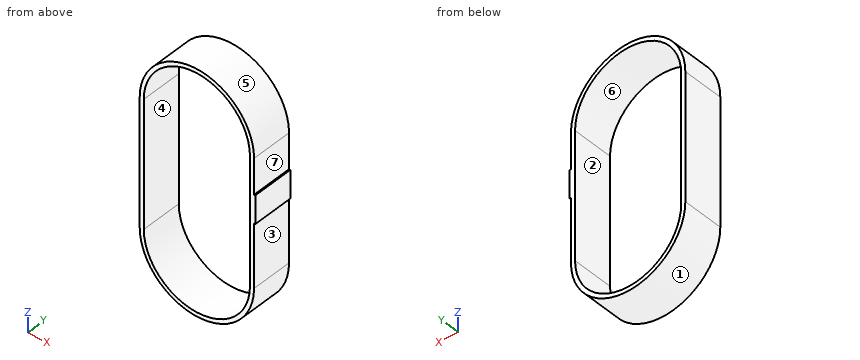
```python
from build123d import *

# Parameters (mm, degrees)
F1_DEPTH = 25.4
F2_T     = -2.54
F3_W     = 25.4
F3_H     = 17.367277
F4_DEPTH = 0.7874


with BuildPart() as f1:
    # F0 (on Front) → F1 (new body)
    with BuildSketch(Plane.XZ):
        with BuildLine():
            ThreePointArc((17.045487, 22.002723), (-18.514513, 57.562723), (-54.074513, 22.002723))
            Line((-54.074513, 22.002723), (-54.074513, -56.737277))
            ThreePointArc((-54.074513, -56.737277), (-18.514513, -92.297277), (17.045487, -56.737277))
            Line((17.045487, -56.737277), (17.045487, 22.002723))
        make_face()
    extrude(amount=F1_DEPTH)

    # F2
    f2_openings = [f1.faces().sort_by_distance(p)[0] for p in [
        (-18.514513, -25.4, -17.367277),
        (-18.514513, 0, -17.367277),
    ]]
    offset(amount=F2_T, openings=f2_openings)

    # F3 (on face) → F4 (join)
    with BuildSketch(Plane.YZ.offset(17.045487)):
        with Locations((-12.7, -8.683638)):
            Rectangle(F3_W, F3_H)
    extrude(amount=F4_DEPTH)


solid = f1.part
```
Here's how the part is built. I have some questions about the finished solid (model axes, mm). Face numbers are marked on the shaded views. A direction names the side the tool comes from. Coordinates: 2 decimals unless noted, no trailing zeros. Loops run counter-clockwise (first coordinate to the right, second up) from the corner with the lowest first, then second, coordinate; pieces in that order, holes last. Notation, with made-up numbers: (35, -25) -> (52, -25) arc R15 cw to (52, -4) -> close; hole circle Ø9 at (82.25, 28). An arc over 180 degrees is marked (long way). Return JSON: item names as keys, results as strings.
1) Will these pins go through, and if not, where does the flat tip stop? pin 1 (4 mm diameter, centred on x = -13.5, y = -23, fed in from +Z); pin 2 (12 mm diameter, centred on y = -21.5, z = -27.5, fed in from +X); pin 3 (3 mm diameter, centred on x = -33, y = -12, fed in from +Z).
Results below:
{"pin 1": "z = 57.43", "pin 2": "x = 17.05", "pin 3": "z = 55.11"}
2) If we section it at C-C, the plane x = -18.5: Write out the boundary of the cut face in (y, z), then the cut area to 3 significant figures.
Results below:
{"outline": "(-25.4, -92.3) -> (0, -92.3) -> (0, -89.76) -> (-25.4, -89.76) -> close; (-25.4, 55.02) -> (0, 55.02) -> (0, 57.56) -> (-25.4, 57.56) -> close", "area": "129 mm²"}
3) I need wall thicknesses on line 1 (X direction, y = -9.75, z = -17); line 2 (X direction, y = -6.25, z = -56); line 3 (Z direction, x = -46, y = -24). Which ranges of each line are inside material? Lowest first, please. Write a range as from..to.
Results below:
{"line 1": "-54.07..-51.53, 14.51..17.83", "line 2": "-54.07..-51.53, 14.51..17.05", "line 3": "-79.3..-75.04, 40.3..44.57"}
4) If we section it at A-A, the plane z = -5.5: Write out the boundary of the cut face in (x, y), then the cut area to 3 significant figures.
Results below:
{"outline": "(-54.07, -25.4) -> (-51.53, -25.4) -> (-51.53, 0) -> (-54.07, 0) -> close; (14.51, -25.4) -> (17.83, -25.4) -> (17.83, 0) -> (14.51, 0) -> close", "area": "149 mm²"}
5) If we section it at B-B, the plane y = -23: Write out the boundary of the cut face in (x, z).
Results below:
{"outline": "(-54.07, -56.74) arc R35.56 ccw to (17.05, -56.74) -> (17.05, -17.37) -> (17.83, -17.37) -> (17.83, 0) -> (17.05, 0) -> (17.05, 22) arc R35.56 ccw to (-54.07, 22) -> close; hole (-51.53, -56.74) arc R33.02 ccw to (14.51, -56.74) -> (14.51, 22) arc R33.02 ccw to (-51.53, 22) -> close"}
6) For the marked faces 1, 2 and 3, which set-ups out of +Z, -Z, +X, -X, +Y, -Y let a thin tool reach every point of the face, with its end or its side?
Results below:
{"face 1": "-Z, +Y, -Y", "face 2": "+Y, -Y", "face 3": "-Z, +X, +Y, -Y"}
7) Thinking about a two-plate mould opening in Z: for the marked faces 4, 5, 6 and 7, which applies, +Z half, -Z half, draft (parallel to the pull), parting line (faces both ways), or undercut?
Results below:
{"face 4": "undercut", "face 5": "+Z half", "face 6": "undercut", "face 7": "draft"}
